Drawing for the job (mm, zero at the part's lowest x, y, z). Give positions to 0.01 mm unless a question says otherwise; leave off trailing zeros. Write each loop counter-clockwise with the first axis right and the second up, starting at its lowest first coordinate (ties: lowest second). Pieces come first, ordered by that corner, then holes. Notation, with made-up numbers: M 45,-16 L 75,-16 A28 cw 75,6 Z; hole C 70,80.5 d5. An arc over 180 degrees is marked long. Write item = value, one per line. Start each with the question number.
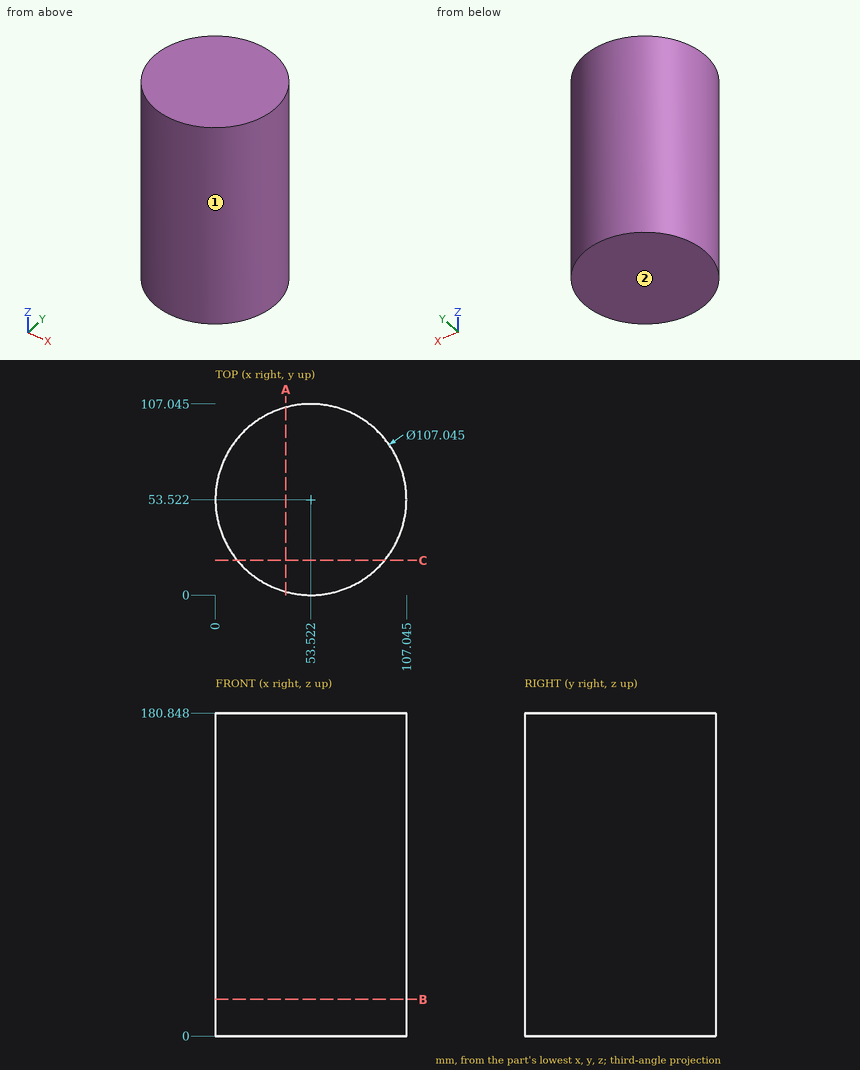
Q1. Probe line 1 along X through (y, z) = (52, 60.5); line 2 along X through (y, z) = (20, 133.5) (1 decimal); line 3 along Y through (x, z) = (14.5, 153.5) (1 decimal). List the from-to ranges inside material, lowest first.
Q2. Slice it at A-A (x = 39.5). Give the cut face in (y, z) (1 decimal), and give its area (3 significant figures).
Q3. Slice it at B-B (z = 20.5). Give the cut face in (x, y) (1 decimal).
Q4. Slice it at C-C (y = 19.5). Give the cut face in (x, z) (1 decimal), and give its area (3 significant figures).
Q5. Two-plate mould, pull along X, no slides. Class the marked faces 1 and 2: +X half, -X half, draft (parallel to the pull), parting line (faces both ways), or undercut.
Q6. Drop flat-ended pins along their axis: P1, Ø1, axis at y = 13.5, z = 76.5, coming from the -X side; P2, Ø5, axis at x = 71.5, z = 20, coming from the +Y side; P3, Ø12, axis at y = 61.5, z = 115, coming from the -X side. Give the stop position or say it passes through.
Working result:
q1.line_1 = 0.02 to 107.02
q1.line_2 = 11.8 to 95.2
q1.line_3 = 16.9 to 90.2
q2.outline = M 1.9,0 L 105.2,0 L 105.2,180.8 L 1.9,180.8 Z
q2.area = 18,700 mm2
q3.outline = C 53.5,53.5 d107
q4.outline = M 12.2,0 L 94.8,0 L 94.8,180.8 L 12.2,180.8 Z
q4.area = 14,900 mm2
q5.face_1 = parting line
q5.face_2 = draft
q6.P1 = 17.43
q6.P2 = 104.76
q6.P3 = 0.04
